CAD build for the part. Positions are in the model's coordinates, mm. A direction names the side the tool comes from. Give positions to 0.01 mm unless a question says otherwise; leave off trailing zeros. Order: outer loops, then holes, each group sorted by start corner. A loop starts at its lowest first (then second) coordinate and runs counter-clockwise, first axis right, second up.
Item 1: Two-plate mould, pull along X, no slides. Class faces 1 (the cylindrical face through (-7.193, 0.751, -0.359)), 2 (the cylindrical face through (-25.351, 27.849, -7.384)), 3 (the cylindrical face through (-25.617, 0.535, -0.172)): released by +X, released by -X, zero draft, split by the parting line, or undercut.
Item 2: Wall check: L1, parallel to X at y = 23, z = 5.5; L2, parallel to X at y = 0.75, z = 0 (1 decimal); L3, parallel to Y at x = -15, z = 7.5. Give the ranges that are in metal, low to high.
Item 3: Band-saw the part on A-A on y = 30.5. Give the cut face in (x, z).
Item 4: Which spindle directions (+Z, -Z, +X, -X, +Y, -Y) get a long thin tool onto all of the face, cutting with end or side? Do faces 4 (the flat face through (-6, 1.524, 0)), 5 (the flat face through (-0.1, 0.5, 12.306)). Say none if no direction does.
Item 5: Band-saw the part on D-D on z = -5.5. Give the cut face in (x, y), plus the area to 3 significant figures.
Item 6: Band-saw the part on B-B on x = 0. Give the cut face in (y, z) (1 decimal).
Item 7: Band-saw the part on C-C on x = 8. Give the cut face in (y, z).
Item 8: Flat gauge pins, fed straight in: P1, Ø9, axis at x = 0, z = 0, coming from the +Y side; P2, Ø1.9, axis at y = 28.58, z = 8.33, coming from the -X side. Where does each tip first touch, or does it go through?
```python
from build123d import *

# Parameters (mm, degrees)
SKETCH1_W               = 49.1998
SKETCH1_H               = 24.6126
SKETCH1_R               = 1.1938
SKETCH1_R_2             = 4.0005
EXTRUDE1_DEPTH          = 1.524
SKETCH1_3_W             = 1.524
SKETCH1_3_H             = 24.6126
EXTRUDE2_DEPTH          = 40.8686
SKETCH4_R               = 4.0005
SKETCH4_R_2             = 1.1938
CUT_EXTRUDE1_DEPTH      = 40.8686
CUT_EXTRUDE1_DEPTH_BACK = 40.8686
FILLET1_R               = 0.254
FILLET2_R               = 1.778


with BuildPart() as part:
    # Sketch1 → Extrude1 (new body)
    with BuildSketch(Plane(origin=(0, 0, 0), x_dir=(1, 0, 0), z_dir=(0, 1, 0))):
        Rectangle(SKETCH1_W, SKETCH1_H)
        with Locations((-8.3312, 0)):
            Circle(SKETCH1_R, mode=Mode.SUBTRACT)
        with Locations((0, -8.3312)):
            Circle(SKETCH1_R, mode=Mode.SUBTRACT)
        Circle(SKETCH1_R_2, mode=Mode.SUBTRACT)
        with Locations((8.3312, 0)):
            Circle(SKETCH1_R, mode=Mode.SUBTRACT)
        with Locations((0, 8.3312)):
            Circle(SKETCH1_R, mode=Mode.SUBTRACT)
    extrude(amount=EXTRUDE1_DEPTH)

    # Sketch1<3> → Extrude2 (add)
    with BuildSketch(Plane(origin=(0, 0, 0), x_dir=(1, 0, 0), z_dir=(0, 1, 0))):
        with Locations((25.3619, 0)):
            Rectangle(SKETCH1_3_W, SKETCH1_3_H)
        with Locations((-25.3619, 0)):
            Rectangle(SKETCH1_3_W, SKETCH1_3_H)
    extrude(amount=EXTRUDE2_DEPTH)

    # Sketch4 → Cut-Extrude1 (cut, two sides)
    with BuildSketch(Plane(origin=(0, 0, 0), x_dir=(0, 0, -1), z_dir=(1, 0, 0))) as cut_extrude1_sk:
        with BuildLine():
            Line((0, 40.8686), (-12.3063, 40.8686))
            Line((-12.3063, 40.8686), (-12.3063, 28.5623))
            ThreePointArc((-12.3063, 28.5623), (-8.701868181, 37.264168181), (0, 40.8686))
        make_face()
        with BuildLine():
            Line((12.3063, 40.8686), (0, 40.8686))
            ThreePointArc((0, 40.8686), (8.701868181, 37.264168181), (12.3063, 28.5623))
            Line((12.3063, 28.5623), (12.3063, 40.8686))
        make_face()
        with Locations((0, 28.575)):
            Circle(SKETCH4_R)
        with Locations((8.3312, 28.575)):
            Circle(SKETCH4_R_2)
        with Locations((0, 36.9062)):
            Circle(SKETCH4_R_2)
        with Locations((-8.3312, 28.575)):
            Circle(SKETCH4_R_2)
        with Locations((0, 20.2438)):
            Circle(SKETCH4_R_2)
    extrude(amount=CUT_EXTRUDE1_DEPTH, mode=Mode.SUBTRACT)
    extrude(cut_extrude1_sk.sketch, amount=-CUT_EXTRUDE1_DEPTH_BACK, mode=Mode.SUBTRACT)

    # Fillet1
    fillet1_edges = [part.edges().sort_by_distance(p)[0] for p in [
        (-24.5999, 1.524, 0),
        (24.5999, 1.524, 0),
    ]]
    fillet(fillet1_edges, radius=FILLET1_R)

    # Fillet2
    fillet2_edges = [part.edges().sort_by_distance(p)[0] for p in [
        (-26.1239, 0, 0),
        (26.1239, 0, 0),
    ]]
    fillet(fillet2_edges, radius=FILLET2_R)


solid = part.part
```
The answers:
1. face 1: undercut
1. face 2: zero draft
1. face 3: released by -X
2. L1: x = -26.12 to -24.6, 24.6 to 26.12
2. L2: x = -25.8 to -9.5, -7.1 to -4, 4 to 7.1, 9.5 to 25.8
2. L3: y = 0 to 1.52
3. outline: (-26.12, -12.15) - (-24.6, -12.15) - (-24.6, -3.51) - (-26.12, -3.51) - close; (-26.12, 3.51) - (-24.6, 3.51) - (-24.6, 12.15) - (-26.12, 12.15) - close; (24.6, -12.15) - (26.12, -12.15) - (26.12, -3.51) - (24.6, -3.51) - close; (24.6, 3.51) - (26.12, 3.51) - (26.12, 12.15) - (24.6, 12.15) - close
4. face 4: +Z, -Z, +Y
4. face 5: +Z, +X, -X, +Y, -Y
5. outline: (-26.12, 1.78) arc R1.78 ccw to (-24.35, 0) - (24.35, 0) arc R1.78 ccw to (26.12, 1.78) - (26.12, 39.57) - (24.6, 39.57) - (24.6, 1.78) arc R0.25 cw to (24.35, 1.52) - (-24.35, 1.52) arc R0.25 cw to (-24.6, 1.78) - (-24.6, 39.57) - (-26.12, 39.57) - close
5. area: 194 mm2
6. outline: (0, -12.3) - (1.5, -12.3) - (1.5, -9.5) - (0, -9.5) - close; (0, -7.1) - (1.5, -7.1) - (1.5, -4) - (0, -4) - close; (0, 4) - (1.5, 4) - (1.5, 7.1) - (0, 7.1) - close; (0, 9.5) - (1.5, 9.5) - (1.5, 12.3) - (0, 12.3) - close
7. outline: (0, -12.31) - (1.52, -12.31) - (1.52, -1.15) - (0, -1.15) - close; (0, 1.15) - (1.52, 1.15) - (1.52, 12.31) - (0, 12.31) - close
8. P1: stops at y = 1.52
8. P2: passes through
